Work out the finished part from the listing and answer in its coordinate system (mm). A direction names the side the tool comes from. Give positions to 0.01 mm unless a question says otherwise; leave off trailing zeros. Order: outer loops, then holes, each group sorted by start corner. A loop starts at its lowest first (then second) coordinate and runs counter-clockwise, first axis right, second up. Notation, with made-up numbers: (18, 27.5) - (60, 27.5) arc R34 cw to (60, 59.5) - close; hole circle Ø1 at (28.5, 46.25). An arc over 180 degrees is marked (long way). Put each result on its own line as item: value.
```python
from build123d import *

# Parameters (mm, degrees)
F2_R     = 5
F5_DEPTH = 2.5


with BuildPart() as f3:
    # F3: sweep along a path in F1
    with BuildLine(Plane.YZ) as f3_path:
        Line((-70, -110), (-70, -10))
        ThreePointArc((-70, -10), (-67.0710678119, -2.9289321881), (-60, 0))
        Line((-60, 0), (0, 0))
    # F0 (on Front) → F3 (sweep)
    with BuildSketch(Plane.XZ):
        with BuildLine():
            Line((-10, 0), (10, 0))
            Line((10, 0), (10, 5))
            Line((10, 5), (5.5, 5))
            ThreePointArc((5.5, 5), (3.3786796564, 5.8786796564), (2.5, 8))
            Line((2.5, 8), (2.5, 32))
            ThreePointArc((2.5, 32), (3.3786796564, 34.1213203436), (5.5, 35))
            Line((5.5, 35), (10, 35))
            Line((10, 35), (10, 40))
            Line((10, 40), (-10, 40))
            Line((-10, 40), (-10, 35))
            Line((-10, 35), (-5.5, 35))
            ThreePointArc((-5.5, 35), (-3.3786796564, 34.1213203436), (-2.5, 32))
            Line((-2.5, 32), (-2.5, 8))
            ThreePointArc((-2.5, 8), (-3.3786796564, 5.8786796564), (-5.5, 5))
            Line((-5.5, 5), (-10, 5))
            Line((-10, 5), (-10, 0))
        make_face()
    sweep(path=f3_path.line)

    # F4: F3 across plane


with BuildPart() as f3_1:
    add(f3.part)
    add(f3.part.mirror(Plane.XZ))

    # F2 (on Right) → F5 (join, symmetric)
    with BuildSketch(Plane.YZ):
        with BuildLine():
            Line((-130, -110), (-100, -110))
            Line((-100, -110), (-100, -40))
            Line((-100, -40), (-142.5800752207, -74.4519548676))
            ThreePointArc((-142.5800752207, -74.4519548676), (-148.8541892248, -96.6722971064), (-130, -110))
        make_face()
        with Locations((-130, -90)):
            Circle(F2_R, mode=Mode.SUBTRACT)
    extrude(amount=F5_DEPTH, both=True)

    # F6: F3 across plane


with BuildPart() as f3_2:
    add(f3_1.part)
    add(f3_1.part.mirror(Plane.XZ))


solid = f3_2.part
```
(1) Section C-C, the plane z = -90 is taken. Count the separate pieces of the cut face and the enclosed holes in it, then the cut area to 3 significant figures.
Geometry check:
separate pieces: 4
enclosed holes: 0
area: 1,020 mm²
(2) Straight lines are drawn through the part: line 1 (Y direction, x = 9, z = -76); line 2 (Y direction, x = 9, z = -5); line 3 (Z direction, x = 6.25, y = -41.5). For each, find the intervals that lie inside material, in ascending order.
Geometry check:
line 1: y = -110 to -105, -75 to -70, 70 to 75, 105 to 110
line 2: y = -109.75 to -104.72, -74.14 to -68.66, 68.66 to 74.14, 104.72 to 109.75
line 3: z = 0 to 5, 35 to 40
(3) Section B-B, the plane y = -40.5 is taken. Write down the section's boundary in (x, z).
Geometry check:
outline: (-10, 0) - (10, 0) - (10, 5) - (5.5, 5) arc R3 cw to (2.5, 8) - (2.5, 32) arc R3 cw to (5.5, 35) - (10, 35) - (10, 40) - (-10, 40) - (-10, 35) - (-5.5, 35) arc R3 cw to (-2.5, 32) - (-2.5, 8) arc R3 cw to (-5.5, 5) - (-10, 5) - close
(4) Given pin 1 (6 mm diameter, centred on x = 0, z = -75, fed in from +Y); pin 2 (12 mm diameter, centred on x = 3, z = -40.5, fed in from +Y); pin 3 (1.3 mm diameter, centred on x = -8, y = -2.5, fed in from -Z); pin 4 (8 mm diameter, centred on y = 130, z = -90, fed in from -X), each flat-ended and moving along its own axis, determine where each tip first touches the part or whether it passes through.
Geometry check:
pin 1: stops at y = 146
pin 2: stops at y = 110
pin 3: stops at z = 0
pin 4: passes through
(5) A tool of negligible diameter and unlimited length cuts with its end or side. For faces 4 (the face through (-7.719, -92.168, 21.468)), 5 (the face through (0.14, 67.15, -3.01)), 6 (the face through (-2.5, 126, -85)), 7 (the face through (5, 110, -59)), 8 (the face through (2.5, -1, 9)), from which of +Z, -Z, +X, -X, +Y, -Y can it reach the whole face along a straight path? Write none if from no direction.
Geometry check:
face 4: -X
face 5: -Z, +X, -X
face 6: +Z, -Z, -X, +Y
face 7: +Z, +Y
face 8: +X
(6) Determine the mould class of faces 1 (the face through (0.035, -126.062, -61.087)), 2 (the face through (0.035, 126.062, -61.087)), 3 (the face through (-7.78, -70.72, 0.49)) for opening direction Y: pulls with the +Y half, pulls with the -Y half, needs draft (parallel to the pull), parting line crosses it, or undercut.
Geometry check:
face 1: pulls with the -Y half
face 2: pulls with the +Y half
face 3: undercut
